```python
from build123d import *

# Parameters (mm, degrees)
BOSS_EXTRUDE1_DEPTH   = 35
SKETCH2_W             = 30
SKETCH2_H             = 28
CUT_EXTRUDE1_DEPTH    = 4.85
SKETCH3_W             = 77.8
SKETCH3_H             = 19
CUT_EXTRUDE2_DEPTH    = 22.35
SKETCH4_W             = 82
SKETCH4_H             = 19.37
CUT_EXTRUDE3_DEPTH    = 29.35
CUT_EXTRUDE5_DEPTH    = 3.08
SKETCH7_W             = 68
SKETCH7_H             = 1.6
CUT_EXTRUDE6_DEPTH    = 26.27
SKETCH8_R             = 2.75
CUT_EXTRUDE7_DEPTH    = 29.35
SKETCH9_R             = 4.75
CUT_EXTRUDE8_DEPTH    = 5.5
M4_TAPPED_HOLE1_D     = 3.3
M4_TAPPED_HOLE1_DEPTH = 8
M4_TAPPED_HOLE1_TIP   = 0.991420021
M4_TAPPED_HOLE2_D     = 3.3
M4_TAPPED_HOLE2_DEPTH = 8
M4_TAPPED_HOLE2_TIP   = 0.991420021
M3_TAPPED_HOLE1_D     = 2.5
M3_TAPPED_HOLE1_DEPTH = 6
M3_TAPPED_HOLE1_TIP   = 0.751075774
M3_TAPPED_HOLE2_D     = 2.5
M3_TAPPED_HOLE2_DEPTH = 6
M3_TAPPED_HOLE2_TIP   = 0.751075774
M3_TAPPED_HOLE3_D     = 2.5
M3_TAPPED_HOLE3_DEPTH = 6
M3_TAPPED_HOLE3_TIP   = 0.751075774
M4_TAPPED_HOLE3_D     = 3.3
M4_TAPPED_HOLE3_DEPTH = 8
M4_TAPPED_HOLE3_TIP   = 0.991420021
SKETCH22_W            = 10
SKETCH22_H            = 30.806567365
CUT_EXTRUDE9_DEPTH    = 0.65


with BuildPart() as part:
    # Sketch1 → Boss-Extrude1 (new body)
    with BuildSketch(Plane.XY):
        Polygon((267.075702076, 27.942429792), (311.075702076, 27.942429792), (311.075702076, 56.292429792), (173.975702076, 56.292429792), (173.975702076, 49.292429792), (143.075702076, 49.292429792), (143.075702076, 47.785708056), (127.075702076, 47.785708056), (127.075702076, 49.292429792), (96.175702076, 49.292429792), (96.175702076, 56.292429792), (-125.924297924, 56.292429792), (-125.924297924, 27.942429792), (233.075702076, 27.942429792), (233.075702076, 42.742429792), (267.075702076, 42.742429792), align=None)
    extrude(amount=BOSS_EXTRUDE1_DEPTH)

    # Sketch2 → Cut-Extrude1 (cut)
    with BuildSketch(Plane(origin=(0, 56.292429792, 0), x_dir=(1, 0, 0), z_dir=(0, 1, 0))):
        with Locations((-47.924297924, -21)):
            Rectangle(SKETCH2_W, SKETCH2_H)
    extrude(amount=-CUT_EXTRUDE1_DEPTH, mode=Mode.SUBTRACT)

    # Sketch3 → Cut-Extrude2 (cut, through all)
    with BuildSketch(Plane(origin=(0, 49.292429792, 0), x_dir=(1, 0, 0), z_dir=(0, 1, 0))):
        with Locations((135.075702076, -9.5)):
            Rectangle(SKETCH3_W, SKETCH3_H)
    extrude(amount=-CUT_EXTRUDE2_DEPTH, mode=Mode.SUBTRACT)

    # Sketch4 → Cut-Extrude3 (cut, through all)
    with BuildSketch(Plane(origin=(0, 56.292429792, 0), x_dir=(1, 0, 0), z_dir=(0, 1, 0))):
        with Locations((250.075702076, -25.315)):
            Rectangle(SKETCH4_W, SKETCH4_H)
    extrude(amount=-CUT_EXTRUDE3_DEPTH, mode=Mode.SUBTRACT)

    # Sketch5 → Cut-Extrude5 (cut)
    with BuildSketch(Plane(origin=(0, 56.292429792, 0), x_dir=(1, 0, 0), z_dir=(0, 1, 0))):
        Polygon((-125.924297924, -6.922171551), (-120.924297924, -4.193432635), (96.175702076, -4.193432635), (173.975702076, -4.193432635), (173.975702076, -6.922171551), (178.975702076, -4.193432635), (306.075702076, -4.193432635), (311.075702076, -6.043688669), (311.075702076, 0), (-125.924297924, 0), align=None)
    extrude(amount=-CUT_EXTRUDE5_DEPTH, mode=Mode.SUBTRACT)

    # Sketch7 → Cut-Extrude6 (cut, through all)
    with BuildSketch(Plane(origin=(0, 53.212429792, 0), x_dir=(1, 0, 0), z_dir=(0, 1, 0))):
        with Locations((250.075702076, -2.13)):
            Rectangle(SKETCH7_W, SKETCH7_H)
    extrude(amount=-CUT_EXTRUDE6_DEPTH, mode=Mode.SUBTRACT)

    # Sketch8 → Cut-Extrude7 (cut, through all)
    with BuildSketch(Plane(origin=(0, 56.292429792, 0), x_dir=(1, 0, 0), z_dir=(0, 1, 0))):
        with Locations((-100.924297924, -25)):
            Circle(SKETCH8_R)
        with Locations((2.075702076, -25)):
            Circle(SKETCH8_R)
        with Locations((184.075702076, -25)):
            Circle(SKETCH8_R)
        with Locations((301.075702076, -25)):
            Circle(SKETCH8_R)
    extrude(amount=-CUT_EXTRUDE7_DEPTH, mode=Mode.SUBTRACT)

    # Sketch9 → Cut-Extrude8 (cut)
    with BuildSketch(Plane(origin=(0, 56.292429792, 0), x_dir=(1, 0, 0), z_dir=(0, 1, 0))):
        with Locations((-100.924297924, -25)):
            Circle(SKETCH9_R)
        with Locations((2.075702076, -25)):
            Circle(SKETCH9_R)
        with Locations((184.075702076, -25)):
            Circle(SKETCH9_R)
        with Locations((301.075702076, -25)):
            Circle(SKETCH9_R)
    extrude(amount=-CUT_EXTRUDE8_DEPTH, mode=Mode.SUBTRACT)

    # M4 Tapped Hole1
    with Locations(Plane(origin=(0, 56.292429792, 0), x_dir=(1, 0, 0), z_dir=(0, 1, 0))):
        with Locations((-116.924297924, -14), (-102.924297924, -14)):
            Hole(M4_TAPPED_HOLE1_D / 2, depth=M4_TAPPED_HOLE1_DEPTH)
            with Locations((0, 0, -(M4_TAPPED_HOLE1_DEPTH + M4_TAPPED_HOLE1_TIP / 2))):  # 118° drill point
                Cone(0, M4_TAPPED_HOLE1_D / 2, M4_TAPPED_HOLE1_TIP, mode=Mode.SUBTRACT)

    # M4 Tapped Hole2
    with Locations(Plane(origin=(0, 49.292429792, 0), x_dir=(1, 0, 0), z_dir=(0, 1, 0))):
        with Locations((105.075702076, -27), (165.075702076, -27)):
            Hole(M4_TAPPED_HOLE2_D / 2, depth=M4_TAPPED_HOLE2_DEPTH)
            with Locations((0, 0, -(M4_TAPPED_HOLE2_DEPTH + M4_TAPPED_HOLE2_TIP / 2))):  # 118° drill point
                Cone(0, M4_TAPPED_HOLE2_D / 2, M4_TAPPED_HOLE2_TIP, mode=Mode.SUBTRACT)

    # M3 Tapped Hole1
    with Locations(Plane(origin=(0, 56.292429792, 0), x_dir=(1, 0, 0), z_dir=(0, 1, 0))):
        with Locations((-16.924297924, -19), (-16.924297924, -28.5), (8.075702076, -9.6), (60.075702076, -9.6), (201.075702076, -9.6), (231.075702076, -9.6), (277.075702076, -9.6), (297.075702076, -9.6)):
            Hole(M3_TAPPED_HOLE1_D / 2, depth=M3_TAPPED_HOLE1_DEPTH)
            with Locations((0, 0, -(M3_TAPPED_HOLE1_DEPTH + M3_TAPPED_HOLE1_TIP / 2))):  # 118° drill point
                Cone(0, M3_TAPPED_HOLE1_D / 2, M3_TAPPED_HOLE1_TIP, mode=Mode.SUBTRACT)

    # M3 Tapped Hole2
    with Locations(Plane.XY.offset(35)):
        with Locations((-54.424297924, 43.292429792), (-41.424297924, 43.292429792), (31.325702076, 48.307679659), (31.325702076, 39.562572504), (41.075702076, 44.894954915), (81.325702076, 51.942429792), (81.325702076, 39.942429792), (164.375702076, 42.742429792), (172.375702076, 42.742429792), (296.075702076, 47.442429792), (306.075702076, 47.442429792)):
            Hole(M3_TAPPED_HOLE2_D / 2, depth=M3_TAPPED_HOLE2_DEPTH)
            with Locations((0, 0, -(M3_TAPPED_HOLE2_DEPTH + M3_TAPPED_HOLE2_TIP / 2))):  # 118° drill point
                Cone(0, M3_TAPPED_HOLE2_D / 2, M3_TAPPED_HOLE2_TIP, mode=Mode.SUBTRACT)

    # M3 Tapped Hole3
    with Locations(Plane.XY.offset(35)):
        with Locations((73.822463361, 53.212429792), (73.822463361, 45.212429792)):
            Hole(M3_TAPPED_HOLE3_D / 2, depth=M3_TAPPED_HOLE3_DEPTH)
            with Locations((0, 0, -(M3_TAPPED_HOLE3_DEPTH + M3_TAPPED_HOLE3_TIP / 2))):  # 118° drill point
                Cone(0, M3_TAPPED_HOLE3_D / 2, M3_TAPPED_HOLE3_TIP, mode=Mode.SUBTRACT)

    # M4 Tapped Hole3
    with Locations(Plane.XY.offset(15.63)):
        with Locations((214.075702076, 51.942429792), (214.075702076, 36.942429792), (286.075702076, 36.942429792), (286.075702076, 51.942429792)):
            Hole(M4_TAPPED_HOLE3_D / 2, depth=M4_TAPPED_HOLE3_DEPTH)
            with Locations((0, 0, -(M4_TAPPED_HOLE3_DEPTH + M4_TAPPED_HOLE3_TIP / 2))):  # 118° drill point
                Cone(0, M4_TAPPED_HOLE3_D / 2, M4_TAPPED_HOLE3_TIP, mode=Mode.SUBTRACT)

    # Sketch22 → Cut-Extrude9 (cut)
    with BuildSketch(Plane(origin=(0, 56.292429792, 0), x_dir=(1, 0, 0), z_dir=(0, 1, 0))):
        with Locations((85.575702076, -19.596716318)):
            Rectangle(SKETCH22_W, SKETCH22_H)
    extrude(amount=-CUT_EXTRUDE9_DEPTH, mode=Mode.SUBTRACT)


solid = part.part
```
The listing builds one solid part. Answer for the finished solid, in the listing's coordinates (mm). A direction names the side the tool comes from. Coordinates: 2 decimals unless noted, no trailing zeros. Answer as a JSON object with one key per item and string values. Group by question number.
1. Determine the mould class of faces 4 (the flat face through (294, 27.942, 13)), 5 (the flat face through (-125.924, 42, 17)), 6 (the flat face through (-98, 50.792, 25)), 7 (the cylindrical face through (1.46, 53.58, 20.29)) for opening direction X: released by +X, released by -X, zero draft, split by the parting line, or undercut.
2. A tool of negligible diameter and unlimited length cuts with its end or side. For faces 1 (the flat face through (-48, 51.442, 21)), 2 (the flat face through (250, 45, 15.63)), 3 (the flat face through (135, 47.786, 27)), from which of +Z, -Z, +X, -X, +Y, -Y can it reach the whole face along a straight path? Write none if from no direction.
3. Flat-ended cylindrical pins translate along their axes: P1, Ø5, axis at x = 88, z = 26.5, coming from the +Y side; P2, Ø1.5, axis at x = 31.33, y = 39.56, coming from the +Z side; P3, Ø3, axis at x = 164.38, y = 42.74, coming from the -Z side. Find the tip coordinate at first contact, or state that the pin passes through.
4. Straight lines are drawn through the part: line 1 (X direction, y = 48.75, z = 31); line 2 (X direction, y = 40.75, z = 7.5); line 3 (X direction, y = 45.5, z = 15.5). For each, find the intervals that lie inside material, in ascending order.
Values follow:
{
 "1": {"face 4": "zero draft", "face 5": "released by -X", "face 6": "undercut", "face 7": "undercut"},
 "2": {"face 1": "+Z, +Y", "face 2": "+Z, +Y, -Y", "face 3": "+Z, -Z, +Y"},
 "3": {"P1": "y = 55.64", "P2": "z = 28.7", "P3": "z = 19"},
 "4": {"line 1": "-125.92 to 30.16, 32.49 to 127.08, 143.08 to 209.08, 291.08 to 311.08", "line 2": "-125.92 to 96.18, 173.98 to 233.08, 267.08 to 311.08", "line 3": "-125.92 to 96.18, 173.98 to 311.08"}
}
